from build123d import *

# Parameters (mm, degrees)
F0_W     = 60
F0_H     = 220
F1_DEPTH = 60
F3_DEPTH = 60.001
F5_DEPTH = 60.0010001
F6_START = -5.46
F4_W     = 55
F4_H     = 26.17
F6_DEPTH = 74.54


with BuildPart() as f1:
    # F0 (on Top) → F1 (new body)
    with BuildSketch(Plane.XY):
        Rectangle(F0_W, F0_H)
    extrude(amount=F1_DEPTH)

    # F2 (on face) → F3 (cut, through all)
    with BuildSketch(Plane.YZ.offset(30)):
        with BuildLine():
            Line((-110, 60), (-110, 5.4592178203))
            add(Edge.make_bspline(
                [(-110, 5.4592178203), (-88.3301750343, 6.2141776062), (-17.4415363661, 7.8038979975), (-2.4796110185, 55.9141440318), (34.855034512, 58.1974692918), (83.83, 60)],
                knots=[0, 0, 0, 0, 0.3774214734, 0.6243161477, 1, 1, 1, 1], degree=3))
            Line((83.83, 60), (-110, 60))
        make_face()
    extrude(amount=-F3_DEPTH, mode=Mode.SUBTRACT)

    # F4 (on face) → F5 (cut, through all)
    with BuildSketch(Plane(origin=(0, 0, 0), x_dir=(1, 0, 0), z_dir=(0, 0, -1))):
        with BuildLine():
            add(Edge.make_bspline(
                [(25.1129814899, -37.9226556811), (26.8734855483, -52.9443126868), (28.4566374792, -68.3794013283), (30, -83.83)],
                knots=[0.8073169996, 0.8073169996, 0.8073169996, 0.8073169996, 1, 1, 1, 1], degree=3))
            Line((30, -83.83), (30, 110))
            Line((30, 110), (-13.4503107729, 110))
            add(Edge.make_bspline(
                [(-13.4503107729, 110), (-10.3085935059, 103.3156568841), (-7.2413287965, 96.6211419831), (-4.3029165498, 89.709023616)],
                knots=[0, 0, 0, 0, 0.1408268689, 0.1408268689, 0.1408268689, 0.1408268689], degree=3))
            add(Edge.make_bspline(
                [(-4.3029165498, 89.709023616), (1.6785085714, 75.6387315772), (7.1260131715, 60.666765223), (11.5807438269, 43.0434755981)],
                knots=[0.1408268689, 0.1408268689, 0.1408268689, 0.1408268689, 0.4274937151, 0.4274937151, 0.4274937151, 0.4274937151], degree=3))
            add(Edge.make_bspline(
                [(11.5807438269, 43.0434755981), (17.4831020937, 19.6932492321), (21.6426160071, -8.3114544361), (25.1129814899, -37.9226556811)],
                knots=[0.4274937151, 0.4274937151, 0.4274937151, 0.4274937151, 0.8073169996, 0.8073169996, 0.8073169996, 0.8073169996], degree=3))
        make_face()
    extrude(amount=-F5_DEPTH, mode=Mode.SUBTRACT)

    # F4 (on face) → F6 (cut)
    with BuildSketch(Plane(origin=(0, 0, 0), x_dir=(1, 0, 0), z_dir=(0, 0, -1)).offset(F6_START)):
        with BuildLine():
            Line((-30, -83.83), (25, -83.83))
            add(Edge.make_bspline(
                [(6.5807438269, 43.0434755981), (15.6026307937, 7.8522057541), (20.3013153969, -37.988897123), (25, -83.83)],
                knots=[0.4274937151, 0.4274937151, 0.4274937151, 0.4274937151, 1, 1, 1, 1], degree=3))
            add(Edge.make_bspline(
                [(-18.4503107729, 110), (-9.3031307537, 89.6604989609), (-0.1559507346, 69.3209979217), (6.5807438269, 43.0434755981)],
                knots=[0, 0, 0, 0, 0.4274937151, 0.4274937151, 0.4274937151, 0.4274937151], degree=3))
            Line((-18.4503107729, 110), (-30, 110))
            Line((-30, 110), (-30, -83.83))
        make_face()
        with Locations((-2.5, -96.915)):
            Rectangle(F4_W, F4_H)
    extrude(amount=-F6_DEPTH, mode=Mode.SUBTRACT)


solid = f1.part
Verification items for the finished model (mm, model axes). A direction names the side the tool comes from. Round coordinates to 2 decimals unless told otherwise and drop trailing zeros. Loops run counter-clockwise (first coordinate to the right, second up) from the corner with the lowest first, then second, coordinate; pieces in that order, holes last. Notation, with made-up numbers: (70.25, 56.25) - (92.25, 56.25) arc R22 cw to (92.25, 94.25) - close; hole circle Ø3 at (23, -37.5). An arc over 180 degrees is marked (long way). Use a Markdown table: item, result. Add a question column.
1. Section check A-A, the plane y = 96. Record the boundary of the cut face in (x, z), plus the area to 3 significant figures.
2. Thickness scan on probe 1 along Z at (x, y) = (23, 80); probe 2 along X at (y, z) = (99.5, 32); probe 3 along X at (y, z) = (73, 47.5). Record the ranges inside material, lowest first. Write a range as [from, to].
3. Gauge pin test, flat ends, axial feed: pin 1 (6 mm diameter, centred on x = -12, y = 73.5, fed in from +Z); pin 2 (1 mm diameter, centred on x = 22, y = 50.5, fed in from +Z); pin 3 (8 mm diameter, centred on y = 94, z = 35.5, fed in from -X). Record the tip position at first contact, or that the pin passes through.
4. Access from +Z, -Z, +X, -X, +Y, -Y to the whole of each face (thin tool, end or side, straight path). Record for faces 1 (the face through (25, 97, 32)), 2 (the face through (-22, -110, 3)).
Checks:
| question | item | result |
|---|---|---|
| 1 | outline | (-30, 0) - (30, 0) - (30, 60) - (25, 60) - (25, 5.46) - (-30, 5.46) - close |
| 1 | area | 600 mm^2 |
| 2 | probe 1 | z = [0, 5.46] |
| 2 | probe 2 | x = [25, 30] |
| 2 | probe 3 | x = [23.89, 28.91] |
| 3 | pin 1 | stops at z = 5.46 |
| 3 | pin 2 | stops at z = 58.51 |
| 3 | pin 3 | stops at x = 25 |
| 4 | face 1 | +Z, -X, +Y |
| 4 | face 2 | +Z, -Z, +X, -X, -Y |
